The listing builds one solid part. Answer for the finished solid, in the listing's coordinates (mm). Face numbers are marked on the shaded views. A direction names the side the tool comes from. Round coordinates to 2 decimals unless told otherwise and drop trailing zeros. Order: outer loops, then holes, each group sorted by start corner. A loop starts at its lowest first (then second) coordinate and runs counter-clockwise, first axis right, second up. Notation, with made-up numbers: (53, 89) - (107, 89) arc R25 cw to (107, 115) - close; hole circle Ø7 at (66.5, -9). An arc over 180 degrees is marked (long way). Write item = value, one per line.
from build123d import *

# Parameters (mm, degrees)
SALIENTE_EXTRUIR1_DEPTH = 4
CROQUIS2_R              = 0.9
SALIENTE_EXTRUIR3_DEPTH = 0.2
SALIENTE_EXTRUIR4_START = -0.2
CROQUIS3_R              = 0.9
SALIENTE_EXTRUIR4_DEPTH = 0.2
CROQUIS4_R              = 0.1
SALIENTE_EXTRUIR5_DEPTH = 1
SALIENTE_EXTRUIR6_START = 1
CROQUIS5_R              = 0.1
SALIENTE_EXTRUIR6_DEPTH = 1


with BuildPart() as part:
    # Croquis1 → Saliente-Extruir1 (new body)
    with BuildSketch(Plane(origin=(0, 0, 0), x_dir=(1, 0, 0), z_dir=(0, 1, 0))):
        with BuildLine():
            Line((18.2, -0.3), (18.2, -1.5))
            Line((18.2, -1.5), (18, -1.5))
            Line((18, -1.5), (18, -0.5))
            ThreePointArc((18, -0.5), (17.853553391, -0.146446609), (17.5, 0))
            Line((17.5, 0), (0, 0))
            Line((0, 0), (0, 0.2))
            Line((0, 0.2), (17.7, 0.2))
            ThreePointArc((17.7, 0.2), (18.053553391, 0.053553391), (18.2, -0.3))
        make_face()
    extrude(amount=SALIENTE_EXTRUIR1_DEPTH)

    # Croquis2 → Saliente-Extruir3 (add)
    with BuildSketch(Plane(origin=(0, 4, 0), x_dir=(1, 0, 0), z_dir=(0, 1, 0))):
        with BuildLine():
            Line((0, 0.2), (3.4, 0.2))
            Line((3.4, 0.2), (3.4, 3.5))
            ThreePointArc((3.4, 3.5), (1.7, 5.2), (0, 3.5))
            Line((0, 3.5), (0, 0.2))
        make_face()
        with Locations(Location((1.7, 3.5, 0), (0, 0, 270))):
            Circle(CROQUIS2_R, mode=Mode.SUBTRACT)
    extrude(amount=-SALIENTE_EXTRUIR3_DEPTH)

    # Croquis3 → Saliente-Extruir4 (add)
    with BuildSketch(Plane(origin=(0, 0, 0), x_dir=(-1, 0, 0), z_dir=(0, -1, 0)).offset(SALIENTE_EXTRUIR4_START)):
        with BuildLine():
            Line((0, 0), (-3.4, 0))
            Line((-3.4, 0), (-3.4, 3.5))
            ThreePointArc((-3.4, 3.5), (-1.7, 5.2), (0, 3.5))
            Line((0, 3.5), (0, 0))
        make_face()
        with Locations(Location((-1.7, 3.5, 0), (0, 0, 270))):
            Circle(CROQUIS3_R, mode=Mode.SUBTRACT)
    extrude(amount=SALIENTE_EXTRUIR4_DEPTH)

    # Croquis4 → Saliente-Extruir5 (add)
    with BuildSketch(Plane(origin=(0, 4, 0), x_dir=(1, 0, 0), z_dir=(0, 1, 0))):
        with Locations(Location((18.1, -1.4, 0), (0, 0, 270))):
            Circle(CROQUIS4_R)
    extrude(amount=SALIENTE_EXTRUIR5_DEPTH)

    # Croquis5 → Saliente-Extruir6 (add)
    with BuildSketch(Plane(origin=(0, 0, 0), x_dir=(-1, 0, 0), z_dir=(0, -1, 0)).offset(SALIENTE_EXTRUIR6_START)):
        with Locations(Location((-18.1, -1.4, 0), (0, 0, 270))):
            Circle(CROQUIS5_R)
    extrude(amount=-SALIENTE_EXTRUIR6_DEPTH)


solid = part.part
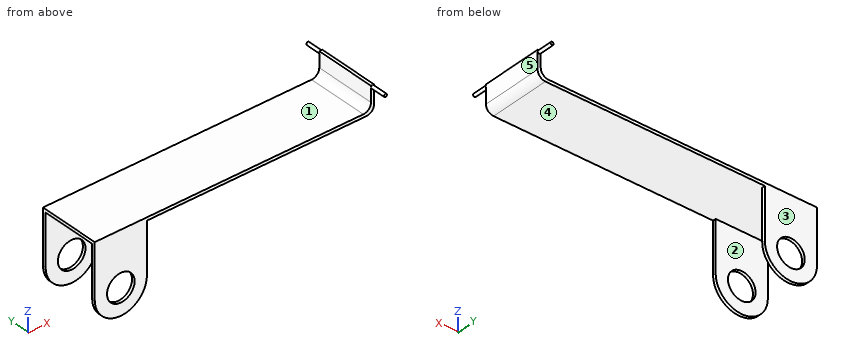
Q1. Section D-D on z = 1 is taken. Determine the outline of the cut face in (x, y), then the cut area to 3 significant figures.
Model answer:
outline = (18, 0) - (18.2, 0) - (18.2, 4) - (18, 4) - close
area = 0.800 mm^2
Q2. Section A-A on z = -1.25 is taken. Determine the outline of the cut face in (x, y).
Model answer:
outline = (0, 0) - (3.4, 0) - (3.4, 0.2) - (0, 0.2) - close; (0, 3.8) - (3.4, 3.8) - (3.4, 4) - (0, 4) - close
Q3. Section B-B on x = 1.7 is taken. Determine the outline of the cut face in (y, z).
Model answer:
outline = (0, -5.2) - (0.2, -5.2) - (0.2, -4.4) - (0, -4.4) - close; (0, -2.6) - (0.2, -2.6) - (0.2, -0.2) - (3.8, -0.2) - (3.8, -2.6) - (4, -2.6) - (4, 0) - (0, 0) - close; (3.8, -5.2) - (4, -5.2) - (4, -4.4) - (3.8, -4.4) - close
Q4. Find the intervals of material crossed by line 1 (Y direction, x = 1.5, z = -1.75); line 2 (Z direction, x = 11.5, y = 2.35); line 3 (X direction, y = 0.1, z = -3.5), in increasing order. Write a range as from..to.
Model answer:
line_1 = 0..0.2, 3.8..4
line_2 = -0.2..0
line_3 = 0..0.8, 2.6..3.4
Q5. For the marked faces 1 and 2, determine the directions among +Z, -Z, +X, -X, +Y, -Y from which every point of the face is accessible in a straight line to the end or side of a thin tool.
Model answer:
face_1 = +Z, -X, +Y, -Y
face_2 = -Z, +X, -X
Q6. Determine the mould class of the marked faces 3, 4 and 5 for opening direction Y: released by +Y, released by -Y, zero draft, split by the parting line, or undercut.
Model answer:
face_3 = released by +Y
face_4 = undercut
face_5 = zero draft
Q7. Section C-C on y = 3.25 is taken. Determine the outline of the cut face in (x, z), then the cut area to 3 significant figures.
Model answer:
outline = (0, -0.2) - (17.7, -0.2) arc R0.5 ccw to (18.2, 0.3) - (18.2, 1.5) - (18, 1.5) - (18, 0.5) arc R0.5 cw to (17.5, 0) - (0, 0) - close
area = 3.94 mm^2
Q8. Flat-ended cylindrical pins translate along their axes: P1, Ø1, axis at x = 2, y = 3.5, coming from the -Z side; P2, Ø2.5, axis at x = 1, z = -2, coming from the -Y side; P3, Ø0.5, axis at y = 1, z = 1, coming from the -X side; P4, Ø2, axis at x = 10, y = 1.5, coming from the -Z side. Find the tip coordinate at first contact, or state that the pin passes through.
Model answer:
P1 = -5.2
P2 = 0
P3 = 18
P4 = -0.2
